The model under review builds one solid part; all positions refer to its coordinate system, in mm. A direction names the side the tool comes from. Give positions to 0.01 mm unless a question says otherwise; leave off trailing zeros. Loops run counter-clockwise (first coordinate to the right, second up) from the corner with the lowest first, then second, coordinate; pieces in that order, holes last. Notation, with made-up numbers: M 6,24 L 47,24 A15 ccw 47,40 Z; hole C -6,51 d7. An arc over 180 degrees is marked long. Put each result on its own line as item: value. Start each with the question number.
Autodesk Inventor part; units mm, degrees
ref_plane "YZ Plane" through (0, 0, 0) normal (1, 0, 0) x (0, 1, 0)
ref_plane "XZ Plane" through (0, 0, 0) normal (0, 1, 0) x (-1, 0, 0)
ref_plane "XY Plane" through (0, 0, 0) normal (0, 0, 1) x (1, 0, 0)
sketch "Sketch1" plane through (0, 0, 0) normal (0, 0, 1) x (1, 0, 0)
  line L0 (-3.9687, 6.8741) -> (3.9687, 6.8741)
  line L1 (3.9687, 6.8741) -> (7.9375, 0)
  line L2 (7.9375, 0) -> (3.9687, -6.8741)
  line L3 (3.9687, -6.8741) -> (-3.9688, -6.8741)
  line L4 (-3.9688, -6.8741) -> (-7.9375, 0)
  line L5 (-7.9375, 0) -> (-3.9687, 6.8741)
  point P0 (0, 0)
  point P1 (0, 6.8741)
  dimension "d0" = 15.875
extrude "Extrusion1" add sketch "Sketch1" along normal blind 6.35
sketch "Sketch2" plane through (0, 0, 6.35) normal (0, 0, 1) x (1, 0, 0)
  circle A0 centre (0, 0) radius 4.7625
  dimension "d3" = 9.525
extrude "Extrusion2" add sketch "Sketch2" along normal blind 177.8
thread "Thread1"
properties part number "7in bolt"
Item 1: Tool access review of faces 1 (the cylindrical face through (-3.78, 2.9, 94.01)), 2 (the flat face through (0, -6.874, 3)): name each direction out of +Z, -Z, +X, -X, +Y, -Y from which nothing blocks a thin tool from reaching the whole face with its end or side.
Item 2: Consider section A-A, the plane x = 0. Write out the cut boundary in (y, z).
Item 3: Consider section C-C, the plane z = 160. Write out the cut boundary in (x, y) (1 decimal).
Item 4: Clearance check with flat-ended pins moving along their axes: pin 1 Ø3 at (x, z) = (-4.5, 103.5) entering from -Y; pin 2 Ø1.5 at (y, z) = (3, 108.5) entering from -X; pin 3 Ø6 at (x, z) = (5, 48.5) entering from -Y. State where each tip first meets the part, or that it passes through.
Item 5: Consider section B-B, the plane y = 3. Write out the cut boundary in (x, z).
Item 6: To check wall thickness, follow L1, parallel to Z at x = -6.75, y = -1; L2, parallel to X at y = 0.5, z = 141.5; L3, parallel to Y at x = -0.25, z = 99.5. State the ranges of each line that lie inside material, in increasing order. Write a range as [from, to].
Report:
1. face 1: +Z
1. face 2: +Z, -Z, +X, -X, -Y
2. outline: M -6.87,0 L 6.87,0 L 6.87,6.35 L 4.76,6.35 L 4.76,184.15 L -4.76,184.15 L -4.76,6.35 L -6.87,6.35 Z
3. outline: C 0,0 d9.5
4. pin 1: y = -3.7
4. pin 2: x = -4.2
4. pin 3: y = -4.32
5. outline: M -6.21,0 L 6.21,0 L 6.21,6.35 L 3.7,6.35 L 3.7,184.15 L -3.7,184.15 L -3.7,6.35 L -6.21,6.35 Z
6. L1: [0, 6.35]
6. L2: [-4.74, 4.74]
6. L3: [-4.76, 4.76]
